CAD build for the part. Positions are in the model's coordinates, mm. A direction names the side the tool comes from. Give positions to 0.01 mm unless a question says otherwise; leave off trailing zeros. Write each loop counter-clockwise with the first axis right and the second up, starting at its lowest first coordinate (ties: lowest second). Pieces come first, ordered by that corner, then holes. Notation, with made-up numbers: (39, 75) - (70, 75) arc R35 cw to (70, 114) - close; hole circle Ø2 at (69.25, 85). An arc over 180 degrees is marked (long way). Answer as a JSON object with one key per item and string values.
Autodesk Inventor part; units mm, degrees
ref_plane "YZ Plane" through (0, 0, 0) normal (1, 0, 0) x (0, 1, 0)
ref_plane "XZ Plane" through (0, 0, 0) normal (0, 1, 0) x (-1, 0, 0)
ref_plane "XY Plane" through (0, 0, 0) normal (0, 0, 1) x (1, 0, 0)
sketch "Sketch1" plane through (0, 0, 0) normal (0, 1, 0) x (-1, 0, 0)
  line L0 (0, 0) -> (35.5, 0)
  line L1 (35.5, 0) -> (35.5, -170)
  line L2 (35.5, -170) -> (0, -170)
  line L3 (0, -170) -> (0, 0)
  dimension "d0" = 35.5
  dimension "d1" = 170
extrude "Extrusion1" add sketch "Sketch1" along normal blind 9
sketch "Sketch2" plane through (0, 9, 0) normal (0, 1, 0) x (1, 0, 0)
  circle A0 centre (-10, 15) radius 3.25 construction
  line L0 (-35.5, 0) -> (0, 0)
  line L1 (0, 0) -> (0, 170)
  line L2 (-13.25, 15) -> (-11.625, 17.8146)
  line L3 (-11.625, 17.8146) -> (-8.375, 17.8146)
  line L4 (-8.375, 17.8146) -> (-6.75, 15)
  line L5 (-6.75, 15) -> (-8.375, 12.1854)
  line L6 (-8.375, 12.1854) -> (-11.625, 12.1854)
  line L7 (-11.625, 12.1854) -> (-13.25, 15)
  circle A1 centre (-10, 150) radius 3.25 construction
  line L8 (-13.25, 150) -> (-11.625, 152.8146)
  line L9 (-11.625, 152.8146) -> (-8.375, 152.8146)
  line L10 (-8.375, 152.8146) -> (-6.75, 150)
  line L11 (-6.75, 150) -> (-8.375, 147.1854)
  line L12 (-8.375, 147.1854) -> (-11.625, 147.1854)
  line L13 (-11.625, 147.1854) -> (-13.25, 150)
  line L14 (0, 170) -> (-35.5, 170)
  circle A2 centre (-10, 15) radius 1.7 construction
  circle A3 centre (-10, 150) radius 1.7 construction
  dimension "d7" = 6.5
  dimension "d10" = 6.5
  dimension "d23" = 135
  dimension "d24" = 15
  dimension "d25" = 10
  dimension "d28" = 3.4
  dimension "d29" = 3.4
extrude "Extrusion2" cut sketch "Sketch2" against normal blind 5
sketch "Sketch3" plane through (0, 0, 0) normal (0, -1, 0) x (1, 0, 0)
  circle A0 centre (-10, -25) radius 3.25 construction
  line L0 (0, 0) -> (-35.5, 0)
  line L1 (-35.5, 0) -> (-35.5, -170)
  line L2 (-11.6286, -27.8125) -> (-13.25, -24.9958)
  line L3 (-13.25, -24.9958) -> (-11.6214, -22.1833)
  line L4 (-11.6214, -22.1833) -> (-8.3714, -22.1875)
  line L5 (-8.3714, -22.1875) -> (-6.75, -25.0042)
  line L6 (-6.75, -25.0042) -> (-8.3786, -27.8167)
  line L7 (-8.3786, -27.8167) -> (-11.6286, -27.8125)
  circle A1 centre (-10, -160) radius 3.25 construction
  line L8 (-6.75, -160) -> (-8.375, -162.8146)
  line L9 (-8.375, -162.8146) -> (-11.625, -162.8146)
  line L10 (-11.625, -162.8146) -> (-13.25, -160)
  line L11 (-13.25, -160) -> (-11.625, -157.1854)
  line L12 (-11.625, -157.1854) -> (-8.375, -157.1854)
  line L13 (-8.375, -157.1854) -> (-6.75, -160)
  line L14 (0, -170) -> (0, 0)
  dimension "d15" = 6.5
  dimension "d18" = 6.5
  dimension "d16" = 25
  dimension "d19" = 135
  dimension "d26" = 10
  dimension "d27" = 10
extrude "Extrusion3" cut sketch "Sketch3" against normal blind 5
sketch "Sketch5" plane through (0, 9, 0) normal (0, 1, 0) x (1, 0, 0)
  circle A0 centre (-10, 15) radius 1.7
  line L0 (0, 0) -> (0, 170)
  line L1 (-35.5, 0) -> (0, 0)
  circle A1 centre (-10, 150) radius 1.7
  circle A2 centre (-10, 25) radius 1.7
  circle A3 centre (-10, 160) radius 1.7
  dimension "d30" = 3.4
  dimension "d31" = 10
  dimension "d32" = 15
  dimension "d33" = 3.4
  dimension "d34" = 10
  dimension "d35" = 135
  dimension "d36" = 3.4
  dimension "d37" = 25
  dimension "d38" = 3.4
  dimension "d39" = 10
  dimension "d40" = 135
extrude "Extrusion4" cut sketch "Sketch5" against normal through all
sketch "Sketch6" plane through (0, 9, 0) normal (0, 1, 0) x (1, 0, 0)
  line L0 (-32.5, 4) -> (-27.7502, 4)
  line L1 (-27.7502, 4) -> (-27.7502, 16.7)
  line L2 (-27.7502, 16.7) -> (-32.5, 16.7)
  line L3 (-32.5, 16.7) -> (-32.5, 4)
  line L4 (-35.5, 0) -> (0, 0)
  line L5 (-35.5, 170) -> (-35.5, 0)
  line L6 (-25.7502, 4) -> (-21.0002, 4)
  line L7 (-21.0002, 4) -> (-21.0002, 16.7)
  line L8 (-21.0002, 16.7) -> (-25.7502, 16.7)
  line L9 (-25.7502, 16.7) -> (-25.7502, 4)
  line L10 (0, 0) -> (0, 170) construction
  line L11 (-35.5, 170) -> (0, 170)
  line L12 (0, 0) -> (-20, 0) construction
  line L13 (-20, 0) -> (-20, 170) construction
  line L14 (-20, 170) -> (0, 170) construction
  line L15 (0, 170) -> (0, 0)
  circle A0 centre (-23.3752, 41.7) radius 1.7
  circle A1 centre (-30.125, 41.7) radius 1.7
  circle A2 centre (-30.125, 49.7) radius 1.7
  circle A3 centre (-23.3752, 49.7) radius 1.7
  dimension "d43" = 4.7498
  dimension "d44" = 12.7
  dimension "d45" = 4
  dimension "d46" = 3
  dimension "d47" = 4.75
  dimension "d48" = 2
  dimension "d49" = 20
  dimension "d50" = 3.4
  dimension "d51" = 25
  dimension "d87" = 3.4
  dimension "d88" = 5.375
  dimension "d90" = 3.4
  dimension "d91" = 8
  dimension "d92" = 3.4
extrude "Extrusion5" cut sketch "Sketch6" against normal through all contours L3 L2 L1 L0 | L9 L8 L7 L6 | A0 | A1 | A2 | A3
sketch "Sketch7" plane through (0, 0, 0) normal (0, -1, 0) x (1, 0, 0)
  circle A0 centre (-23.3752, -41.7) radius 1.7
  circle A1 centre (-23.3752, -41.7) radius 3.25 construction
  line L0 (-23.3752, -38.45) -> (-20.5606, -40.075)
  line L1 (-20.5606, -40.075) -> (-20.5606, -43.325)
  line L2 (-20.5606, -43.325) -> (-23.3752, -44.95)
  line L3 (-23.3752, -44.95) -> (-26.1898, -43.325)
  line L4 (-26.1898, -43.325) -> (-26.1898, -40.075)
  line L5 (-26.1898, -40.075) -> (-23.3752, -38.45)
  circle A2 centre (-30.1625, -41.7) radius 3.25 construction
  line L6 (-30.125, -38.4502) -> (-27.3294, -40.1076)
  line L7 (-27.3294, -40.1076) -> (-27.3669, -43.3574)
  line L8 (-27.3669, -43.3574) -> (-30.2, -44.9498)
  line L9 (-30.2, -44.9498) -> (-32.9956, -43.2924)
  line L10 (-32.9956, -43.2924) -> (-32.9581, -40.0426)
  line L11 (-32.9581, -40.0426) -> (-30.125, -38.4502)
  point P0 (0, 0)
  dimension "d89" = 6.5
  dimension "d54" = 6.5
extrude "Extrusion6" cut sketch "Sketch7" against normal blind 5
sketch "Sketch8" plane through (-35.5, 0, -170) normal (-1, 0, 0) x (0, 0, 1)
  circle A0 centre (159.65, 4.5) radius 1.4605
  line L0 (0, 9) -> (170, 9)
  line L1 (170, 0) -> (170, 9)
  dimension "d57" = 2.921
  dimension "d58" = 4.5
  dimension "d59" = 10.35
hole "Hole1" at (-35.5, 4.5, -10.35) direction (1, 0, 0) diameter 2.921 depth 21 counterbore diameter 3.4 counterbore depth 1.5
sketch "Sketch9" plane through (-21.0002, 9, -16.7) normal (-1, 0, 0) x (0, 0, 1)
  circle A0 centre (6.35, -4.5) radius 1.4605
  circle A1 centre (6.35, -4.5) radius 2.54
  point P0 (16.7, -9)
  dimension "d67" = 5.08
extrude "Extrusion7" add sketch "Sketch9" along normal blind 0.2032
sketch "Sketch10" plane through (-27.7502, 9, -16.7) normal (-1, 0, 0) x (0, 0, 1)
  circle A0 centre (6.35, -4.5) radius 1.7
  circle A1 centre (6.35, -4.5) radius 2.54
  point P0 (16.7, -9)
  dimension "d70" = 5.08
extrude "Extrusion8" add sketch "Sketch10" along normal blind 0.2032
sketch "Sketch11" plane through (-25.7502, 9, -4) normal (1, 0, 0) x (0, 0, -1)
  circle A0 centre (6.35, -4.5) radius 1.7
  circle A1 centre (6.35, -4.5) radius 2.54
  point P0 (-4, -9)
  dimension "d73" = 5.08
extrude "Extrusion9" add sketch "Sketch11" along normal blind 0.2032
sketch "Sketch12" plane through (-32.5, 9, -4) normal (1, 0, 0) x (0, 0, -1)
  circle A0 centre (6.35, -4.5) radius 1.7
  circle A1 centre (6.35, -4.5) radius 2.54
  point P0 (-4, -9)
  dimension "d76" = 5.08
extrude "Extrusion10" add sketch "Sketch12" along normal blind 0.2032
sketch "Sketch14" plane through (0, 0, -170) normal (0, 0, -1) x (-1, 0, 0)
  circle A0 centre (18, 4.5) radius 2.25
  line L0 (35.5, 0) -> (0, 0)
  line L1 (0, 0) -> (0, 9)
  dimension "d82" = 4.5
  dimension "d83" = 4.5
  dimension "d84" = 18
extrude "Extrusion11" cut sketch "Sketch14" against normal blind 71
sketch "Sketch15" plane through (0, 9, 0) normal (0, 1, 0) x (1, 0, 0)
  circle A0 centre (-30.125, 49.7) radius 1.7
  circle A1 centre (-30.125, 49.7) radius 3.25 construction
  circle A2 centre (-23.3752, 49.7) radius 1.7
  circle A3 centre (-23.3752, 49.7) radius 3.25 construction
  line L0 (-30.125, 46.45) -> (-32.9396, 48.075)
  line L1 (-32.9396, 48.075) -> (-32.9396, 51.325)
  line L2 (-32.9396, 51.325) -> (-30.125, 52.95)
  line L3 (-30.125, 52.95) -> (-27.3104, 51.325)
  line L4 (-27.3104, 51.325) -> (-27.3104, 48.075)
  line L5 (-27.3104, 48.075) -> (-30.125, 46.45)
  line L6 (-23.3752, 46.45) -> (-26.1898, 48.075)
  line L7 (-26.1898, 48.075) -> (-26.1898, 51.325)
  line L8 (-26.1898, 51.325) -> (-23.3752, 52.95)
  line L9 (-23.3752, 52.95) -> (-20.5606, 51.325)
  line L10 (-20.5606, 51.325) -> (-20.5606, 48.075)
  line L11 (-20.5606, 48.075) -> (-23.3752, 46.45)
  point P0 (0, 0)
  dimension "d93" = 6.5
  dimension "d94" = 6.5
extrude "Extrusion12" cut sketch "Sketch15" against normal blind 5
ref_plane "Work Plane3" through (0, 4.5, 0) normal (0, 1, 0) x (1, 0, 0)
properties part number "Front fixed bottom coupler"
(1) Flat gauge pins, fed straight in: P1, Ø3.5, axis at y = 4.5, z = -10.35, coming from the -X side; P2, Ø3, axis at x = -9.5, z = -159, coming from the -Y side; P3, Ø1.7, axis at y = 4.5, z = -11, coming from the -X side; P4, Ø2.5, axis at x = -23.38, z = -49.7, coming from the +Y side. Where does each tip first touch, or does it go through?
Answer key:
{"P1": "stops at x = -35.5", "P2": "stops at y = 5", "P3": "stops at x = -34", "P4": "passes through"}
(2) Pull direction Z, two halves, no side cores. Call faces 4 (the face through (-35.5, 4, -84)), 5 (the face through (-8.6, 5, -158.7)): pulls with the +Z half, pulls with the -Z half, needs draft (parallel to the pull), parting line crosses it, or undercut.
Answer key:
{"face 4": "needs draft", "face 5": "undercut"}
(3) Probe L1, parallel to Z at x = -10, y = 7.4; L2, parallel to X at y = 2.4, z = -49.7 (3 decimals); L3, parallel to Z at x = -12, y = 1.5. List the from-to ranges inside material, lowest first. Write a range as [from, to].
Answer key:
{"L1": "z = [-170, -161.7], [-158.3, -152.81], [-147.19, -26.7], [-23.3, -17.81], [-12.19, 0]", "L2": "x = [-35.5, -31.825], [-28.425, -25.075], [-21.675, 0]", "L3": "z = [-170, -162.17], [-157.83, -27.17], [-22.84, 0]"}
(4) Saw through at B-B, the plane x = -10. State how many separate pieces and enclosed holes the cut face has, and give its area (3 significant figures).
Answer key:
{"separate pieces": "5", "enclosed holes": "0", "area": "1,360 mm²"}
(5) 3-axis set-ups, long thin cutter, end or side, ignore diameter. For faces 1 (the face through (-28.76, 2.46, -44.14)), 2 (the face through (-12.426, 6.535, -13.573)), 3 (the face through (-23, 5, -16.7)): which of +Z, -Z, +X, -X, +Y, -Y reach the whole face in a straight line?
Answer key:
{"face 1": "-Y", "face 2": "+Y", "face 3": "+Y, -Y"}
(6) Saw through at A-A, the plane z = -120. Give the cut face in (x, y).
Answer key:
{"outline": "(-35.5, 0) - (0, 0) - (0, 9) - (-35.5, 9) - close; hole circle Ø4.5 at (-18, 4.5)"}
